Model file for the job. Use its own axes, mm. Face numbers are marked on the shaded views. A direction names the side the tool comes from. Give positions to 0.01 mm unless a question says otherwise; leave off trailing zeros. Loops run counter-clockwise (first coordinate to the right, second up) from the corner with the lowest first, then second, coordinate; pieces in that order, holes last. Notation, with made-up numbers: M -24.5,11.25 L -7.5,11.25 A28 cw -7.5,43.25 Z; hole C 1,8 d9. An arc over 180 degrees is marked long. Answer in a Markdown table with one row per item.
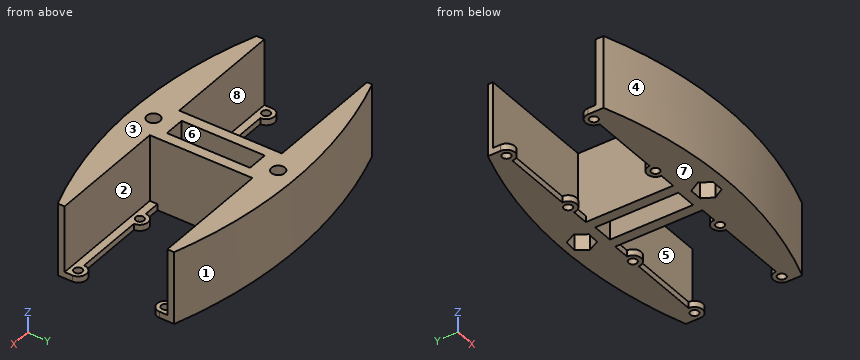
```python
from build123d import *

# Parameters (mm, degrees)
SKETCH_R        = 1
PAD_DEPTH       = 1.5
PAD001_DEPTH    = 16
SKETCH002_R     = 1.6
POCKET_DEPTH    = 30
POCKET001_DEPTH = 14
SKETCH004_W     = 5
SKETCH004_H     = 20
POCKET002_DEPTH = 20


with BuildPart() as part:
    # Sketch → Pad (new body)
    with BuildSketch(Plane.XY):
        with BuildLine():
            Line((13, 10.5), (30, 10.5))
            ThreePointArc((30, 10.5), (32, 8.5), (34, 10.5))
            Line((34, 10.5), (34, 14))
            ThreePointArc((34, 14), (-0.033512, 19.410124), (-34, 13.594018))
            Line((-34, 10.5), (-34, 13.594018))
            ThreePointArc((-34, 10.5), (-32, 8.5), (-30, 10.5))
            Line((-13, 10.5), (-30, 10.5))
            ThreePointArc((-13, 10.5), (-11, 8.5), (-9, 10.5))
            Line((-9, 10.5), (-5, 10.5))
            Line((-5, 10.5), (-5, -10.5))
            Line((-5, -10.5), (-9, -10.5))
            ThreePointArc((-9, -10.5), (-11, -8.5), (-13, -10.5))
            Line((-13, -10.5), (-30, -10.5))
            ThreePointArc((-30, -10.5), (-32, -8.5), (-34, -10.5))
            Line((-34, -10.5), (-34, -14.265938))
            ThreePointArc((-34, -14.265938), (0.023508, -20.143886), (34, -14))
            Line((34, -10.5), (34, -14))
            ThreePointArc((34, -10.5), (32, -8.5), (30, -10.5))
            Line((13, -10.5), (30, -10.5))
            ThreePointArc((13, -10.5), (11, -8.5), (9, -10.5))
            Line((5, -10.5), (9, -10.5))
            Line((5, 10.5), (5, -10.5))
            Line((9, 10.5), (5, 10.5))
            ThreePointArc((9, 10.5), (11, 8.5), (13, 10.5))
        make_face()
        with Locations((11, 10.5)):
            Circle(SKETCH_R, mode=Mode.SUBTRACT)
        with Locations((11, -10.5)):
            Circle(SKETCH_R, mode=Mode.SUBTRACT)
        with Locations((32, 10.5)):
            Circle(SKETCH_R, mode=Mode.SUBTRACT)
        with Locations((32, -10.5)):
            Circle(SKETCH_R, mode=Mode.SUBTRACT)
        with Locations((-11, 10.5)):
            Circle(SKETCH_R, mode=Mode.SUBTRACT)
        with Locations((-11, -10.5)):
            Circle(SKETCH_R, mode=Mode.SUBTRACT)
        with Locations((-32, 10.5)):
            Circle(SKETCH_R, mode=Mode.SUBTRACT)
        with Locations((-32, -10.5)):
            Circle(SKETCH_R, mode=Mode.SUBTRACT)
    extrude(amount=PAD_DEPTH)

    # Sketch001 → Pad001 (new body)
    with BuildSketch(Plane.XY.offset(1.5)):
        with BuildLine():
            Line((-34, 12.35), (-5, 12.35))
            Line((-5, 12.35), (-5, 10.5))
            Line((-5, 10.5), (-5, -10.5))
            Line((-5, -10.5), (-5, -12.35))
            Line((-34, -12.35), (-5, -12.35))
            Line((-34, -12.35), (-34, -14.265938))
            ThreePointArc((-34, -14.265938), (0.023508, -20.143886), (34, -14))
            Line((34, -12.35), (34, -14))
            Line((34, -12.35), (5, -12.35))
            Line((5, -10.5), (5, -12.35))
            Line((5, 10.5), (5, -10.5))
            Line((5, 12.35), (5, 10.5))
            Line((34, 12.35), (5, 12.35))
            Line((34, 12.35), (34, 14))
            ThreePointArc((34, 14), (-0.033512, 19.410124), (-34, 13.594018))
            Line((-34, 13.594018), (-34, 12.35))
        make_face()
    extrude(amount=PAD001_DEPTH)

    # Sketch002 → Pocket (cut)
    with BuildSketch(Plane(origin=(0, 0, 0), x_dir=(1, 0, 0), z_dir=(0, 0, -1))):
        with Locations((0, 15)):
            Circle(SKETCH002_R)
        with Locations((0, -15)):
            Circle(SKETCH002_R)
    extrude(amount=-POCKET_DEPTH, mode=Mode.SUBTRACT)

    # Sketch003 → Pocket001 (cut)
    with BuildSketch(Plane(origin=(0, 0, 0), x_dir=(1, 0, 0), z_dir=(0, 0, -1))):
        Polygon((1.491232, 12.396881), (2.999983, 14.989885), (1.508751, 17.593004), (-1.491232, 17.603119), (-2.999983, 15.010115), (-1.508751, 12.406996), align=None)
        Polygon((1.360539, -17.673749), (2.995804, -15.158613), (1.635265, -12.484864), (-1.360539, -12.326251), (-2.995804, -14.841387), (-1.635265, -17.515136), align=None)
    extrude(amount=-POCKET001_DEPTH, mode=Mode.SUBTRACT)

    # Sketch004 → Pocket002 (cut)
    with BuildSketch(Plane.XY.offset(17.5)):
        Rectangle(SKETCH004_W, SKETCH004_H)
    extrude(amount=-POCKET002_DEPTH, mode=Mode.SUBTRACT)


solid = part.part
```
(1) Wall check: L1, parallel to Y at x = 0, z = 16.5; L2, parallel to X at y = -9.5, z = 12.5; L3, parallel to Z at x = 29, y = -11.5. Give the ranges that are in metal, low to high.
Established:
| item | result |
|---|---|
| L1 | y = -20.14 to -16.6, -13.4 to -10, 10 to 13.4, 16.6 to 19.41 |
| L2 | x = -5 to -2.5, 2.5 to 5 |
| L3 | z = 0 to 1.5 |
(2) Flat gauge pins, fed straight in: P1, Ø1.6, axis at x = 19.5, z = 1, coming from the +Y side; P2, Ø1.2, axis at x = -23.5, z = 0.5, coming from the +Y side; P3, Ø10, axis at x = -18.5, z = 14, coming from the -Y side. Where does each tip first touch, or does it go through?
Established:
| item | result |
|---|---|
| P1 | stops at y = 17.85 |
| P2 | stops at y = 16.77 |
| P3 | stops at y = -19.27 |
(3) Saw through at B-B, the plane z = 14.75. Give the cut face in (x, y).
Established:
| item | result |
|---|---|
| outline | M -34,-14.27 A99.16 ccw 34,-14 L 34,-12.35 L 5,-12.35 L 5,12.35 L 34,12.35 L 34,14 A105.78 ccw -34,13.59 L -34,12.35 L -5,12.35 L -5,-12.35 L -34,-12.35 Z; hole M -2.5,-10 L 2.5,-10 L 2.5,10 L -2.5,10 Z; hole C 0,-15 d3.2; hole C 0,15 d3.2 |
(4) Saw through at C-C, the plane x = -11. Give the cut face in (y, z).
Established:
| item | result |
|---|---|
| outline | M -19.57,0 L -11.5,0 L -11.5,1.5 L -12.35,1.5 L -12.35,17.5 L -19.57,17.5 Z; M -9.5,0 L -8.5,0 L -8.5,1.5 L -9.5,1.5 Z; M 8.5,0 L 9.5,0 L 9.5,1.5 L 8.5,1.5 Z; M 11.5,0 L 18.77,0 L 18.77,17.5 L 12.35,17.5 L 12.35,1.5 L 11.5,1.5 Z |
(5) Which spindle directions (+Z, -Z, +X, -X, +Y, -Y) get a long thin tool onto all of the face, cutting with end or side? Do the marked faces 5, 6, 7 and 8. Say none if no direction does.
Established:
| item | result |
|---|---|
| face 5 | +Z, +X |
| face 6 | +Z, -Z |
| face 7 | -Z, +X, -X, +Y, -Y |
| face 8 | +Z, -X |
(6) Saw through at D-D, the plane z = 11.25. Give the cut face in (x, y).
Established:
| item | result |
|---|---|
| outline | M -34,-14.27 A99.16 ccw 34,-14 L 34,-12.35 L 5,-12.35 L 5,12.35 L 34,12.35 L 34,14 A105.78 ccw -34,13.59 L -34,12.35 L -5,12.35 L -5,-12.35 L -34,-12.35 Z; hole M -3,-15.01 L -1.49,-17.6 L 1.51,-17.59 L 3,-14.99 L 1.49,-12.4 L -1.51,-12.41 Z; hole M -3,14.84 L -1.36,12.33 L 1.64,12.48 L 3,15.16 L 1.36,17.67 L -1.64,17.52 Z; hole M -2.5,-10 L 2.5,-10 L 2.5,10 L -2.5,10 Z |
(7) Mould opens along Y. For the marked faces 1, 2, 3 and 4 say: pulls with the +Y half, pulls with the -Y half, needs draft (parallel to the pull), parting line crosses it, or undercut.
Established:
| item | result |
|---|---|
| face 1 | pulls with the +Y half |
| face 2 | undercut |
| face 3 | needs draft |
| face 4 | pulls with the -Y half |
(8) Saw through at A-A, the plane y = 5. Give the cut face in (x, z).
Established:
| item | result |
|---|---|
| outline | M -5,0 L -2.5,0 L -2.5,17.5 L -5,17.5 Z; M 2.5,0 L 5,0 L 5,17.5 L 2.5,17.5 Z |
